Answer from the drawing. Dimensions are ordinates in mm from the lowest x, y and z of the part. Coordinates: 2 decimals unless noted, no trailing zeros. Write each loop counter-clockwise with the first axis right and the second up, starting at its lowest first coordinate (ties: lowest second). Pieces come first, ordered by that corner, then holes. Notation, with made-up numbers: (40, -1.5) -> (89, -1.5) arc R16 ccw to (89, 7.5) -> close; hole circle Ø5 at (34.25, 63). An arc over 180 degrees is marked (long way). One line per item, written item: value. Start each with the question number.
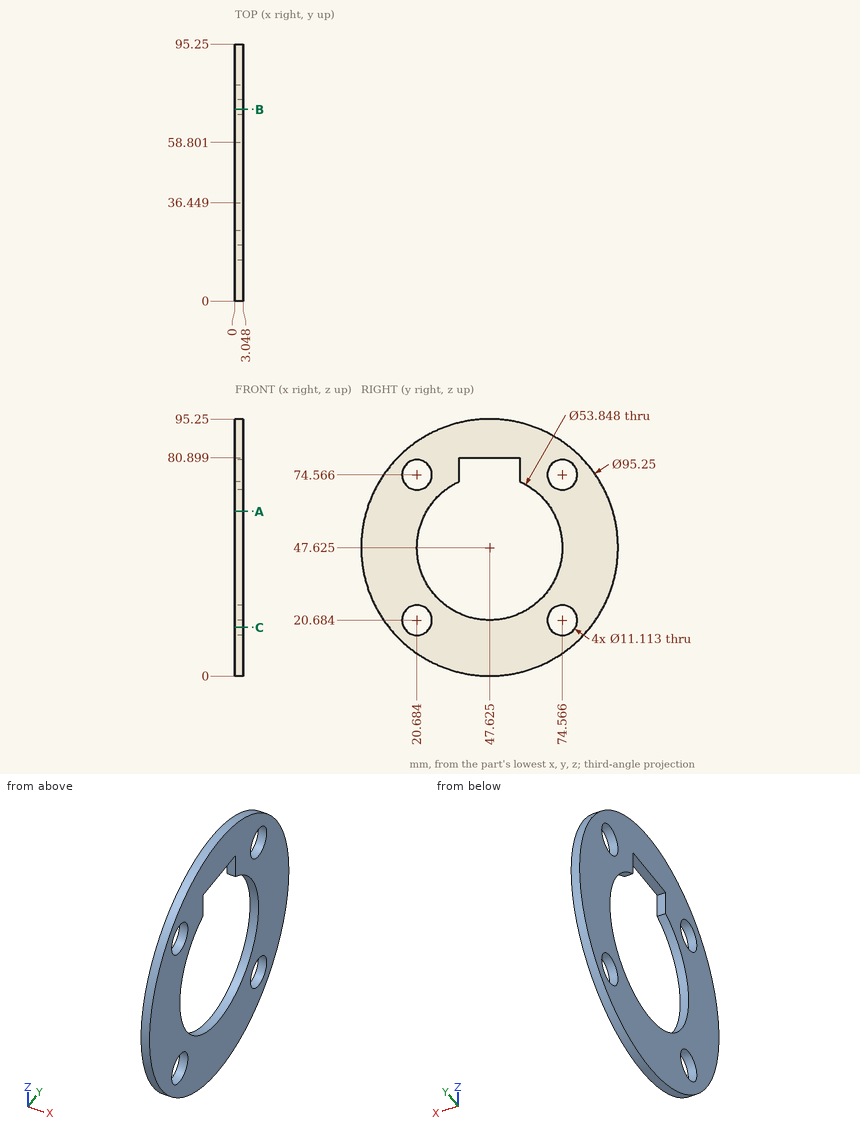
1. A cutting plane is placed at A-A on z = 61. Give the vertices of the cut face in (x, y), then the cut area to 3 significant figures.
2. Find the intervals of material crossed by probe 1 along Z at (x, y) = (2, 24) (1 decimal); probe 2 along Z at (x, y) = (2.55, 47) (1 decimal); probe 3 along Z at (x, y) = (2.25, 44.5), in increasing order. Write a range as from..to.
3. A cutting plane is placed at B-B on y = 71. Give the vertices of the cut face in (x, z) (1 decimal).
4. Given pin 1 (10 mm diameter, centred on y = 74.57, z = 20.68, fed in from -X); pin 2 (0.9 mm diameter, centred on x = 2, z = 76.5, fed in from -Y), each flat-ended and moving along its own axis, determine where each tip first touches the part or whether it passes through.
5. A cutting plane is placed at C-C on z = 18. Count the separate pieces of the cut face and the enclosed holes in it, then the cut area to 3 significant figures.
Derived:
1. outline: (0, 1.92) -> (3.05, 1.92) -> (3.05, 24.26) -> (0, 24.26) -> close; (0, 70.99) -> (3.05, 70.99) -> (3.05, 93.33) -> (0, 93.33) -> close
1. area: 136 mm2
2. probe 1: z = 6.3..16.2, 25.1..34.7, 60.5..70.1, 79..89
2. probe 2: z = 0..20.7, 80.9..95.2
2. probe 3: z = 0.1..20.88, 80.9..95.15
3. outline: (0, 6.1) -> (3, 6.1) -> (3, 16.4) -> (0, 16.4) -> close; (0, 24.9) -> (3, 24.9) -> (3, 34.3) -> (0, 34.3) -> close; (0, 61) -> (3, 61) -> (3, 70.3) -> (0, 70.3) -> close; (0, 78.8) -> (3, 78.8) -> (3, 89.1) -> (0, 89.1) -> close
4. pin 1: passes through
4. pin 2: stops at y = 9.41
5. separate pieces: 3
5. enclosed holes: 0
5. area: 168 mm2
